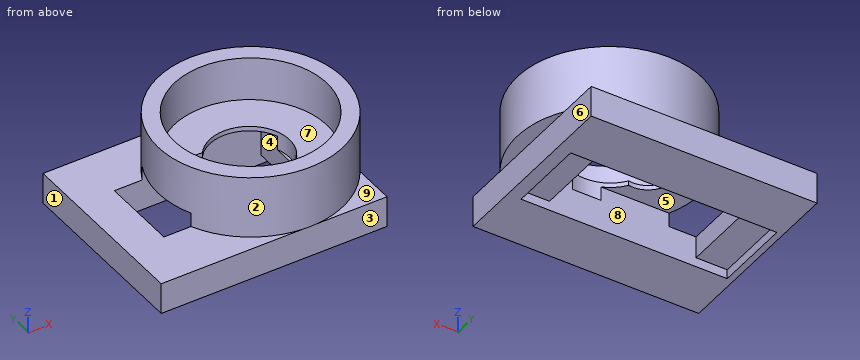
```python
from build123d import *

# Parameters (mm, degrees)
ESQUISSE1_W             = 36.200001836
ESQUISSE1_H             = 29.499999305
BOSS_EXTRU_1_DEPTH      = 5
ESQUISSE2_W             = 33.052998595
ESQUISSE2_H             = 12.371999211
ENL_V_MAT_EXTRU_1_DEPTH = 5
BOSS_EXTRU_2_START      = 5
ESQUISSE3_W             = 4.558359629
ESQUISSE3_H             = 12.371999211
ESQUISSE3_W_2           = 4.999999888
ESQUISSE3_H_2           = 12.380001135
BOSS_EXTRU_2_DEPTH      = 3.5
BOSS_EXTRU_7_START      = 5
ESQUISSE5_R             = 14.763664953
ESQUISSE5_R_2           = 12.203597673
BOSS_EXTRU_7_DEPTH      = 10
BOSS_EXTRU_5_DEPTH      = 2
BOSS_EXTRU_5_DEPTH_BACK = 1
BOSS_EXTRU_5_START      = 6
ESQUISSE4_R             = 12.398139185
ENL_V_MAT_EXTRU_3_REACH = 53.128
ESQUISSE6_W             = 2.256513492
ESQUISSE6_H             = 12.371999211


with BuildPart() as part:
    # Esquisse1 → Boss.-Extru.1 (new body)
    with BuildSketch(Plane.XY):
        with Locations((5.10000065, -15.249999676)):
            Rectangle(ESQUISSE1_W, ESQUISSE1_H)
    extrude(amount=BOSS_EXTRU_1_DEPTH)

    # Esquisse2 → Enlèv. mat.-Extru.1 (cut)
    with BuildSketch(Plane.XY):
        with Locations((4.523499403, -15.158999246)):
            Rectangle(ESQUISSE2_W, ESQUISSE2_H)
    extrude(amount=ENL_V_MAT_EXTRU_1_DEPTH, mode=Mode.SUBTRACT)

    # Esquisse3 → Boss.-Extru.2 (add)
    with BuildSketch(Plane.XY.offset(BOSS_EXTRU_2_START)):
        with Locations((18.770818887, -15.158999246)):
            Rectangle(ESQUISSE3_W, ESQUISSE3_H)
        with Locations((-9.50299995, -15.163000208)):
            Rectangle(ESQUISSE3_W_2, ESQUISSE3_H_2)
    extrude(amount=-BOSS_EXTRU_2_DEPTH)

    # Esquisse5 → Boss.-Extru.7 (add)
    with BuildSketch(Plane.XY.offset(BOSS_EXTRU_7_START)):
        with Locations(Location((10.794645366, -15.275821527, 0), (0, 0, 204.273249948))):
            Circle(ESQUISSE5_R)
        with Locations(Location((10.794645366, -15.275821527, 0), (0, 0, 209.823305738))):
            Circle(ESQUISSE5_R_2, mode=Mode.SUBTRACT)
    extrude(amount=BOSS_EXTRU_7_DEPTH)

    # Esquisse4 → Boss.-Extru.5 (add, two sides: drawn at the far end of the back side and taken through both)
    with BuildSketch(Plane.XY.offset(BOSS_EXTRU_5_START - BOSS_EXTRU_5_DEPTH_BACK)):
        with Locations((10.5484362, -15.38812394)):
            Circle(ESQUISSE4_R)
        with BuildLine():
            ThreePointArc((5.299216058, -19.01722353), (16.929328279, -15.482422447), (5.408748548, -11.605494329))
            ThreePointArc((5.408748548, -11.605494329), (0.800592824, -15.244067738), (5.299216058, -19.01722353))
        make_face(mode=Mode.SUBTRACT)
    extrude(amount=BOSS_EXTRU_5_DEPTH + BOSS_EXTRU_5_DEPTH_BACK)

    # Enlèv. mat.-Extru.3: up to this face of the body (flat: up to its plane)
    enl_v_mat_extru_3_end = Plane(part.part.faces().sort_by_distance((16.491639072, -15.158999246, 3.25))[0])
    # Esquisse6 → Enlèv. mat.-Extru.3 (cut, up to the picked face)
    with BuildSketch(Plane.ZY.offset(13.000000268), mode=Mode.PRIVATE) as enl_v_mat_extru_3_sk1:
        with Locations((6.128256634, -15.158999246)):
            Rectangle(ESQUISSE6_W, ESQUISSE6_H)
    enl_v_mat_extru_3_tool1 = split(extrude(enl_v_mat_extru_3_sk1.sketch, amount=-ENL_V_MAT_EXTRU_3_REACH, mode=Mode.PRIVATE), bisect_by=enl_v_mat_extru_3_end, keep=Keep.BOTH, mode=Mode.PRIVATE)
    add(enl_v_mat_extru_3_tool1.solids().sort_by(Axis((-13, -15.158999, 6.128257), (1, 0, 0)))[0], mode=Mode.SUBTRACT)


solid = part.part
```
The listing builds one solid part. Answer for the finished solid, in the listing's coordinates (mm). Face numbers are marked on the shaded views. A direction names the side the tool comes from. Coordinates: 2 decimals unless noted, no trailing zeros. Write each loop counter-clockwise with the first axis right and the second up, starting at its lowest first coordinate (ties: lowest second). Pieces come first, ordered by that corner, then holes.
Q1. Which of the six approach directions +Z, -Z, +X, -X, +Y, -Y give full straight-line access (tool end or side, diameter ignored) to the marked faces 5, 6, 7, 8 and 9?
Returned:
face 5: -Z, -X
face 6: -Z, +X, +Y, -Y
face 7: +Z
face 8: -Z
face 9: +Z, +X, -Y
Q2. Section B-B, the plane y = -15.3 is taken. Write down the section's boundary in (x, z), then the cut area to 3 significant figures.
Returned:
outline: (-13, 0) - (-12, 0) - (-12, 1.5) - (-7, 1.5) - (-7, 5) - (-13, 5) - close; (-3.97, 7.26) - (0.8, 7.26) - (0.8, 8) - (-1.41, 8) - (-1.41, 15) - (-3.97, 15) - close; (16.49, 1.5) - (21.05, 1.5) - (21.05, 0) - (23.2, 0) - (23.2, 5) - (25.56, 5) - (25.56, 15) - (23, 15) - (23, 5) - (22.95, 5) - (22.95, 8) - (16.93, 8) - (16.93, 5) - (16.49, 5) - close
area: 114 mm2
Q3. Section A-A, the plane x = -6.5 is taken. Write down the section's boundary in (y, z) (3 decimals), then the cut area to 3 significant figures.
Returned:
outline: (-30, 0) - (-21.345, 0) - (-21.345, 5) - (-30, 5) - close; (-8.973, 0) - (-0.5, 0) - (-0.5, 5) - (-8.973, 5) - close
area: 85.6 mm2
Q4. Given P1, Ø12, axis at x = 16, y = -18, coming from the +Z side; P2, Ø8.5, axis at x = 19.5, y = -12.5, coming from the +Z side; P3, Ø5, axis at y = -7.5, z = 10.5, coming from the +X side; P4, Ø1.9, axis at x = 25, y = -12.5, coming from the -Z side, each flat-ended and moving along its own axis, determine where each tip first touches the part or whether it passes through.
Returned:
P1: stops at z = 8
P2: stops at z = 15
P3: stops at x = 24.58
P4: stops at z = 5
Q5. Find the intervals of material crossed by line 1 along X through (y, z) = (-20, 1); line 2 along X through (y, z) = (-15, 9); line 3 along Y through (x, z) = (0.5, 1.75) (3 decimals), in increasing order.
Returned:
line 1: x = -13 to -12, 21.05 to 23.2
line 2: x = -3.97 to -1.41, 23 to 25.56
line 3: y = -30 to -21.345, -8.973 to -0.5
Q6. The mould has two halves that part along Y. Classify the marked faces 1, 2, 3 and 4: released by +Y, released by -Y, zero draft, split by the parting line, or undercut.
Returned:
face 1: zero draft
face 2: split by the parting line
face 3: released by -Y
face 4: undercut
Q7. Section D-D, the plane z = 10.5 is taken. Write down the section's boundary in (x, y) (3 decimals), then the cut area to 3 significant figures.
Returned:
outline: circle Ø29.527 at (10.795, -15.276); hole circle Ø24.407 at (10.795, -15.276)
area: 217 mm2
Q8. Section C-C, the plane y = -6.25 is taken. Write down the section's boundary in (x, z).
Returned:
outline: (-13, 0) - (23.2, 0) - (23.2, 5) - (22.48, 5) - (22.48, 15) - (19.01, 15) - (19.01, 5) - (18.93, 5) - (18.93, 8) - (2.58, 8) - (2.58, 15) - (-0.89, 15) - (-0.89, 5) - (-13, 5) - close
